```python
from build123d import *

# Parameters (mm, degrees)
SKETCH1_W                        = 9.525
SKETCH1_H                        = 72.39
BOSS_EXTRUDE1_DEPTH              = 9.525
F_18_0_1695_DIAMETER_HOLE1_D     = 4.3053
F_18_0_1695_DIAMETER_HOLE1_DEPTH = 15.24
F_18_0_1695_DIAMETER_HOLE1_TIP   = 1.293442612
CUT_EXTRUDE1_REACH               = 11.525


with BuildPart() as part:
    # Sketch1 → Boss-Extrude1 (new body)
    with BuildSketch(Plane(origin=(0, 0, 0), x_dir=(1, 0, 0), z_dir=(0, 1, 0))):
        with Locations((-20.976080696, -16.361756412)):
            Rectangle(SKETCH1_W, SKETCH1_H)
    extrude(amount=BOSS_EXTRUDE1_DEPTH)

    # #18 (0.1695) Diameter Hole1
    with Locations(Plane(origin=(0, 9.525, 0), x_dir=(-1, 0, 0), z_dir=(0, 1, 0))):
        with Locations((20.976080696, 43.944568912)):
            Hole(F_18_0_1695_DIAMETER_HOLE1_D / 2, depth=F_18_0_1695_DIAMETER_HOLE1_DEPTH)
            with Locations((0, 0, -(F_18_0_1695_DIAMETER_HOLE1_DEPTH + F_18_0_1695_DIAMETER_HOLE1_TIP / 2))):  # 118° drill point
                Cone(0, F_18_0_1695_DIAMETER_HOLE1_D / 2, F_18_0_1695_DIAMETER_HOLE1_TIP, mode=Mode.SUBTRACT)

    # Sketch4 → Cut-Extrude1 (cut, up to next)
    with BuildSketch(Plane(origin=(0, 9.525, 0), x_dir=(1, 0, 0), z_dir=(0, 1, 0)), mode=Mode.PRIVATE) as cut_extrude1_sk1:
        with BuildLine():
            Line((-18.9306781, 11.856056088), (-18.9306781, 10.586056088))
            ThreePointArc((-18.9306781, 10.586056088), (-20.976080696, 8.540653493), (-23.021483291, 10.586056088))
            Line((-23.021483291, 10.586056088), (-23.021483291, 11.856056088))
            ThreePointArc((-23.021483291, 11.856056088), (-20.976080696, 13.901458684), (-18.9306781, 11.856056088))
        make_face()
    cut_extrude1_tool1 = extrude(cut_extrude1_sk1.sketch, amount=-CUT_EXTRUDE1_REACH, mode=Mode.PRIVATE) & part.part
    add(cut_extrude1_tool1.solids().sort_by_distance((-20.976081, 9.525, -11.221056))[0], mode=Mode.SUBTRACT)


solid = part.part
```
For this review, take the finished solid that the model builds, in its own axes (mm). A direction names the side the tool comes from. Coordinates: 2 decimals unless noted, no trailing zeros. Loops run counter-clockwise (first coordinate to the right, second up) from the corner with the lowest first, then second, coordinate; pieces in that order, holes last.
1. Insertion check: P1, Ø3.5, axis at x = -20.98, z = 43.94, coming from the -Y side. The pin has a flat end and moves straight along its axis. Give the tip position at first contact, or say it passes through.
2. Add section A-A, the plane y = 7.75. Give the boundary of the cut face in (x, z).
3. For line 1 (Z direction, x = -20.75, y = 9); line 2 (Z direction, x = -22.75, y = 3.5); line 3 (X direction, y = 8, z = 45), list the stretches that pass through material, from the lowest coordinate up.
4. Mouldability with a two-part tool opening along X and no side actions: class faces 3 (the flat face through (-21, 5, 52.557)), 4 (the cylindrical face through (-19.983, 4.696, 42.035)), 5 (the flat face through (-16.214, 5, 17)) as +X half, -X half, draft (parallel to the pull), parting line (faces both ways), or undercut.
5. Add section B-B, the plane x = -22. Give the boundary of the cut face in (y, z) (3 decimals).
6. For faces 1 (the cylindrical face through (-21, 4.8, -13.9)), 2 (the flat face through (-21, 0, 16)), list the 3-axis set-ups (+Z, -Z, +X, -X, +Y, -Y) from which the entire face can be reached by the end or side of a thin tool; tool diameter is ignored.
Result:
1. P1: passes through
2. outline: (-25.74, -19.83) - (-16.21, -19.83) - (-16.21, 52.56) - (-25.74, 52.56) - close; hole circle Ø4.31 at (-20.98, 43.94); hole (-23.02, -11.86) arc R2.05 ccw to (-18.93, -11.86) - (-18.93, -10.59) arc R2.05 ccw to (-23.02, -10.59) - close
3. line 1: z = -19.83 to -13.89, -8.55 to 41.8, 46.09 to 52.56
3. line 2: z = -19.83 to -12.87, -9.57 to 42.73, 45.16 to 52.56
3. line 3: x = -25.74 to -22.85, -19.1 to -16.21
4. face 3: draft
4. face 4: undercut
4. face 5: +X half
5. outline: (0, -19.833) - (9.525, -19.833) - (9.525, -13.627) - (0, -13.627) - close; (0, -8.815) - (9.525, -8.815) - (9.525, 42.051) - (0, 42.051) - close; (0, 45.838) - (9.525, 45.838) - (9.525, 52.557) - (0, 52.557) - close
6. face 1: +Y, -Y
6. face 2: +Z, -Z, +X, -X, -Y
